```python
from build123d import *

# Parameters (mm, degrees)
BOSS_EXTRUDE1_DEPTH  = 58
SKETCH3_R            = 11
CUT_EXTRUDE1_DEPTH   = 13
SKETCH4_R            = 8
CUT_EXTRUDE2_DEPTH   = 89.820042783
SKETCH5_R            = 15
CUT_EXTRUDE3_DEPTH   = 35
SKETCH6_W            = 30
SKETCH6_H            = 29
CUT_EXTRUDE4_DEPTH   = 35
M5_TAPPED_HOLE1_D    = 4.2
SKETCH12_W           = 20
SKETCH12_H           = 58
CUT_EXTRUDE6_DEPTH   = 38
M8_CLEARANCE_HOLE1_D = 9


with BuildPart() as part:
    # Sketch2 → Boss-Extrude1 (new body)
    with BuildSketch(Plane(origin=(0, 0, 0), x_dir=(1, 0, 0), z_dir=(0, 1, 0))):
        Polygon((-50, 0), (0, 0), (50, 0), (50, 58), (-50, 58), align=None)
    extrude(amount=BOSS_EXTRUDE1_DEPTH)

    # Sketch3 → Cut-Extrude1 (cut)
    with BuildSketch(Plane.XY.offset(-58)):
        with Locations(Location((0, 29, 0), (0, 0, 180))):
            Circle(SKETCH3_R)
    extrude(amount=CUT_EXTRUDE1_DEPTH, mode=Mode.SUBTRACT)

    # Sketch4 → Cut-Extrude2 (cut, through all)
    with BuildSketch(Plane(origin=(0, 0, -45), x_dir=(-1, 0, 0), z_dir=(0, 0, -1))):
        with Locations((0, 29)):
            Circle(SKETCH4_R)
    extrude(amount=-CUT_EXTRUDE2_DEPTH, mode=Mode.SUBTRACT)

    # Sketch5 → Cut-Extrude3 (cut)
    with BuildSketch(Plane.XY):
        with Locations((0, 29)):
            Circle(SKETCH5_R)
    extrude(amount=-CUT_EXTRUDE3_DEPTH, mode=Mode.SUBTRACT)

    # Sketch6 → Cut-Extrude4 (cut)
    with BuildSketch(Plane.XY):
        with Locations((0, 43.5)):
            Rectangle(SKETCH6_W, SKETCH6_H)
    extrude(amount=-CUT_EXTRUDE4_DEPTH, mode=Mode.SUBTRACT)

    # M5 Tapped Hole1 (through all)
    with Locations(Plane(origin=(8.704435936, 17.394887918, 0), x_dir=(1, 0, 0), z_dir=(0, 0, 1))):
        with Locations((16.044301406, 36.353849424), (-33.453173277, 36.353849424), (-33.453173277, -13.143625259), (16.044301406, -13.143625259)):
            Hole(M5_TAPPED_HOLE1_D / 2)

    # Sketch12 → Cut-Extrude6 (cut)
    with BuildSketch(Plane(origin=(0, 58, 0), x_dir=(1, 0, 0), z_dir=(0, 1, 0))):
        with Locations((-40, 29)):
            Rectangle(SKETCH12_W, SKETCH12_H)
        with Locations((40, 29)):
            Rectangle(SKETCH12_W, SKETCH12_H)
    extrude(amount=-CUT_EXTRUDE6_DEPTH, mode=Mode.SUBTRACT)

    # M8 Clearance Hole1 (through all)
    with Locations(Plane(origin=(8.704435936, 20, -505.336111538), x_dir=(1, 0, 0), z_dir=(0, 1, 0))):
        with Locations((-48.704435936, -458.836111538), (-48.704435936, -493.836111538), (31.295564064, -458.836111538), (31.295564064, -493.836111538), (-48.704435936, 58.078352635), (31.295564064, 58.078352635)):
            Hole(M8_CLEARANCE_HOLE1_D / 2)


solid = part.part
```
Geometry check sheet. Reference: the model listing, model coordinates, mm. A direction names the side the tool comes from. Give positions to 0.01 mm unless a question says otherwise; leave off trailing zeros. Loops run counter-clockwise (first coordinate to the right, second up) from the corner with the lowest first, then second, coordinate; pieces in that order, holes last. Notation, with made-up numbers: M 38,1 L 46,1 A20 ccw 46,12 Z; hole C 48.5,37.25 d5. An arc over 180 degrees is marked long. Answer as CSV lines item,"result".
Item 1: Cross-section at A-A on x = 0. Record the cut outline in (y, z).
Values:
outline,"M 0,-58 L 18,-58 L 18,-45 L 21,-45 L 21,-35 L 14,-35 L 14,0 L 0,0 Z; M 37,-45 L 40,-45 L 40,-58 L 58,-58 L 58,-35 L 37,-35 Z"
Item 2: Depth check by flat-ended pin: P1, Ø3, axis at y = 22, z = -51.5, coming from the +X side; P2, Ø16, axis at x = -42, z = -39, coming from the +Y side; P3, Ø9.5, axis at x = 0, y = 29, coming from the -Z side; P4, Ø9, axis at x = 3, y = 35, coming from the +Z side. Enter the tip coordinate at first touch or a pass-through.
Values:
P1,"stops at x = 30"
P2,"stops at y = 20"
P3,"passes through"
P4,"stops at z = -35"
Item 3: Access from +Z, -Z, +X, -X, +Y, -Y to the whole of each face (thin tool, end or side, straight path). Record for faces 5 (the flat face through (0, 41, -35)), 6 (the flat face through (-40, 20, -29)), 7 (the flat face through (2, 37, -45)).
Values:
face 5,"+Z, +Y"
face 6,"+Z, -Z, -X, +Y"
face 7,"-Z"
Item 4: Release check for a two-part mould opening along X. For faces 1 (the flat face through (-30, 39, -29)), 2 (the flat face through (30, 39, -29)), 3 (the flat face through (40, 20, -29)), 4 (the cylindrical face through (37.92, 9.86, -42.51)) record: pulls with the +X half, pulls with the -X half, needs draft (parallel to the pull), parting line crosses it, or undercut.
Values:
face 1,"pulls with the -X half"
face 2,"pulls with the +X half"
face 3,"needs draft"
face 4,"undercut"
Item 5: Cross-section at B-B on x = -40. Record the cut outline in (y, z).
Values:
outline,"M 0,-58 L 20,-58 L 20,-51 L 0,-51 Z; M 0,-42 L 20,-42 L 20,-16 L 0,-16 Z; M 0,-7 L 20,-7 L 20,0 L 0,0 Z"
Item 6: Material ranges on line 1 (Z direction, x = 40, y = 12.5); line 2 (X direction, y = 49, z = -10.5); line 3 (X direction, y = 54, z = -22.5), recorded low to high.
Values:
line 1,"z = -58 to -51, -42 to -16, -7 to 0"
line 2,"x = -30 to -15, 15 to 30"
line 3,"x = -30 to -26.83, -22.66 to -15, 15 to 22.66, 26.83 to 30"
Item 7: Cross-section at C-C on y = 11. Record the cut outline in (x, z), and give its area (3 significant figures).
Values:
outline,"M -50,-58 L 50,-58 L 50,0 L -50,0 Z; hole C -40,-46.5 d9; hole C -40,-11.5 d9; hole C 40,-46.5 d9; hole C 40,-11.5 d9"
area,"5,550 mm²"
Item 8: Cross-section at D-D on y = 31.5. Record the cut outline in (x, z), and give its area (3 significant figures).
Values:
outline,"M -30,-58 L -10.71,-58 L -10.71,-45 L -7.6,-45 L -7.6,-35 L -15,-35 L -15,0 L -30,0 Z; M 7.6,-45 L 10.71,-45 L 10.71,-58 L 30,-58 L 30,0 L 15,0 L 15,-35 L 7.6,-35 Z"
area,"2,000 mm²"
